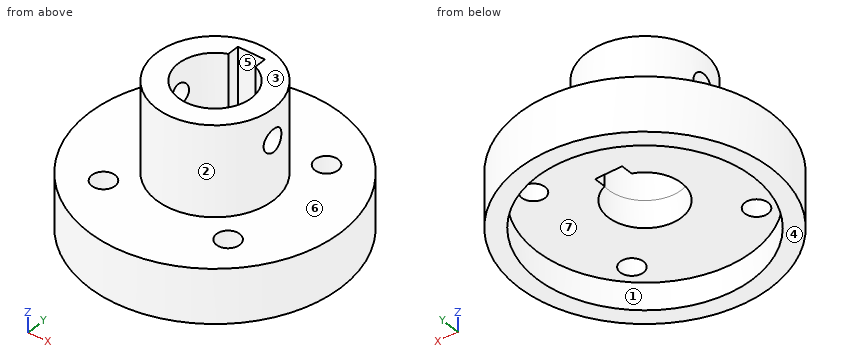
Autodesk Inventor part; units mm, degrees
ref_plane "YZ Plane" through (0, 0, 0) normal (1, 0, 0) x (0, 1, 0)
ref_plane "XZ Plane" through (0, 0, 0) normal (0, 1, 0) x (-1, 0, 0)
ref_plane "XY Plane" through (0, 0, 0) normal (0, 0, 1) x (1, 0, 0)
sketch "Hub" plane through (0, 0, 0) normal (0, 0, 1) x (1, 0, 0)
  circle A0 centre (0, 0) radius 6.6 construction
  circle A1 centre (-6.9148, 6.9148) radius 1.5875 construction
  circle A2 centre (6.9148, 6.9148) radius 1.5875 construction
  circle A3 centre (-6.9148, -6.9148) radius 1.5875 construction
  circle A4 centre (6.9148, -6.9148) radius 1.5875 construction
  line L0 (-6.9148, 6.9148) -> (6.9148, 6.9148) construction
  line L1 (6.9148, 6.9148) -> (6.9148, -6.9148) construction
  line L2 (6.9148, -6.9148) -> (-6.9148, -6.9148) construction
  line L3 (-6.9148, -6.9148) -> (-6.9148, 6.9148) construction
  circle A5 centre (0, 0) radius 12.958 construction
  line L4 (-6.9148, -6.9148) -> (6.9148, 6.9148) construction
  line L5 (-6.9148, 6.9148) -> (-5.7923, 5.7923) construction
  line L6 (-5.7923, 5.7923) -> (-4.6669, 4.6669) construction
  line L7 (-8.0373, 8.0373) -> (-9.1627, 9.1627) construction
  circle A6 centre (0, 0) radius 4.0625
  line L8 (0, 4.0625) -> (0, 5.1125) construction
  line L9 (0, -21.9812) -> (0, 19.9969) construction
  line L10 (-1.5, 5.1125) -> (1.5, 5.1125)
  line L11 (-1.5, 5.1125) -> (-1.5, 3.7754)
  line L12 (1.5, 5.1125) -> (1.5, 3.7754)
  circle A7 centre (0, 0) radius 14
  circle A8 centre (6.9148, 6.9148) radius 1.2891
  circle A9 centre (6.9148, -6.9148) radius 1.2891
  circle A10 centre (-6.9148, -6.9148) radius 1.2891
  circle A11 centre (-6.9148, 6.9148) radius 1.2891
  circle A12 centre (6.9148, -6.9148) radius 2.84 construction
  circle A13 centre (12.3744, -12.3744) radius 1.621 construction
  circle A14 centre (12.3744, -12.3744) radius 3.61 construction
  dimension "d0" = 13.2
  dimension "d1" = 3.175
  dimension "d5" = 13.8296
  dimension "d6" = 45
  dimension "d9" = 8.125
  dimension "d10" = 1.05
  dimension "d11" = 3
  dimension "d21" = 2.5781
  dimension "d27" = 28
  dimension "d34" = 5.68
  dimension "d35" = 7.22
extrude "HubFeature" add sketch "Hub" against normal blind 6
sketch "Lip" plane through (0, 0, 0) normal (0, 0, 1) x (1, 0, 0)
  circle A0 centre (0, 0) radius 6.5
  arc A1 (-1.5, 3.7754) -> (1.5, 3.7754) centre (0, 0) ccw
  line L0 (1.5, 5.1125) -> (1.5, 3.7754)
  line L1 (-1.5, 5.1125) -> (1.5, 5.1125)
  line L2 (-1.5, 3.7754) -> (-1.5, 5.1125)
  dimension "d28" = 13
extrude "LipFeature" add sketch "Lip" along normal blind 10
sketch "SetScrewHole" plane through (0, 0, 0) normal (1, 0, 0) x (0, 1, 0)
  line L0 (6.5, 10) -> (-6.5, 10) construction
  line L1 (0, 10) -> (0, 0) construction
  circle A0 centre (0, 6.5) radius 1.25
  dimension "d30" = 2.5
  dimension "d31" = 3.5
extrude "SetScrewHoleFeature" cut sketch "SetScrewHole" along normal through all both and the other way through all
sketch "Sketch7" plane through (0, 0, -6) normal (0, 0, -1) x (-1, 0, 0)
  circle A0 centre (0, 0) radius 14
  circle A1 centre (0, 0) radius 12
  dimension "d38" = 24
extrude "Extrusion6" cut sketch "Sketch7" against normal blind 3 contours A1
properties part number "BaseHub"
Can you work these out from the model? Positions are in its coordinate system, mm. Face numbers are marked on the shaded views. A direction names the side the tool comes from. Round coordinates to 2 decimals unless told otherwise and drop trailing zeros. Write each loop counter-clockwise with the first axis right and the second up, starting at its lowest first coordinate (ties: lowest second). Pieces come first, ordered by that corner, then holes. Notation, with made-up numbers: M 72,88 L 98,88 A21 cw 98,109 Z; hole C 56,57 d7. An arc over 180 degrees is marked long. Use CSV: the item, a comma, the result in double quotes.
(1) We'd pull the mould along X, two halves only. Please class the marked faces 1, 2 and 3: +X half, -X half, draft (parallel to the pull), parting line (faces both ways), or undercut.
Check values:
face 1,"undercut"
face 2,"parting line"
face 3,"draft"
(2) On a 3-axis mill with a long thin cutter (end or side, diameter ignored), from which of +Z, -Z, +X, -X, +Y, -Y can I reach the whole of each face in a straight line? I mean the marked faces 4, 5, 6 and 7. Say none if no direction works.
Check values:
face 4,"-Z, +X, -X, +Y, -Y"
face 5,"+Z, -Z"
face 6,"+Z"
face 7,"-Z"
(3) I need wall thicknesses on line 1 along Y through (x, z) = (0, -4.8); line 2 along Y through (x, z) = (-0.25, 8); line 3 along X through (y, z) = (-0.25, 8.5). Which ranges of each line are inside material? Lowest first, please.
Check values:
line 1,"-14 to -12, 12 to 14"
line 2,"-6.5 to -4.05, 5.11 to 6.5"
line 3,"-6.5 to -4.05, 4.05 to 6.5"
(4) Imagine slicing it at C-C (z = 0.75). Write out the boundary of the cut face in (x, y).
Check values:
outline,"C 0,0 d13; hole M -1.5,3.78 A4.06 ccw long 1.5,3.78 L 1.5,5.11 L -1.5,5.11 Z"
(5) I'm going to push flat-ended pins straight in: pin 1 (7 mm diameter, centred on x = -4, y = 2, fed in from -Z); pin 2 (0.7 mm diameter, centred on y = 4.5, z = 1.5, fed in from -X); pin 3 (3.5 mm diameter, centred on x = -0.5, z = 2.5, fed in from -Y). Where does each tip first touch, or does it pass through?
Check values:
pin 1,"z = -3"
pin 2,"x = -5"
pin 3,"y = -6.5"
(6) Imagine slicing it at D-D (z = 6.5). Write out the boundary of the cut face in (x, y).
Check values:
outline,"M -6.38,-1.25 A6.5 ccw 6.38,-1.25 L 3.87,-1.25 A4.06 cw -3.87,-1.25 Z; M -6.38,1.25 L -3.87,1.25 A4.06 cw -1.5,3.78 L -1.5,5.11 L 1.5,5.11 L 1.5,3.78 A4.06 cw 3.87,1.25 L 6.38,1.25 A6.5 ccw Z"
(7) Imagine slicing it at B-B (x = 6). Write out the boundary of the cut face in (y, z).
Check values:
outline,"M -12.65,-6 L -10.39,-6 L -10.39,-3 L -7.82,-3 L -7.82,0 L -12.65,0 Z; M -6.01,-3 L 6.01,-3 L 6.01,0 L 2.5,0 L 2.5,10 L -2.5,10 L -2.5,0 L -6.01,0 Z; M 7.82,-3 L 10.39,-3 L 10.39,-6 L 12.65,-6 L 12.65,0 L 7.82,0 Z; hole C 0,6.5 d2.5"
